Verification items for the finished model (mm, model axes). Face numbers are marked on the shaded views. A direction names the side the tool comes from. Give positions to 0.01 mm unless a question says otherwise; leave off trailing zeros. Order: outer loops, then holes, each group sorted by start corner. A loop starts at its lowest first (then second) coordinate and runs counter-clockwise, first axis right, second up. Notation, with made-up numbers: (8, -12.75) -> (45, -12.75) arc R12 cw to (45, 0.25) -> close; hole circle Ø10 at (-17, -12). An arc over 180 degrees is marked (long way). Return JSON: item names as keys, results as strings. Group by question number.
(1) Cross-section at C-C on y = 67.5. Enter the section's corners in (x, z).
(2) Tool access check on the marked faces 1, 2 and 3. Record the directions out of +Z, -Z, +X, -X, +Y, -Y that give a thin tool (end or side, any length) a straight path to the whole face; none if there is none.
(3) Thickness scan on line 1 along Y through (x, z) = (-35.5, 1.7); line 2 along X through (y, z) = (-35, 2); line 3 along Y through (x, z) = (30, 46). Record the ranges inside material, lowest first.
(4) Cross-section at D-D on x = 35.5. Enter the section's corners in (y, z).
(5) Cross-section at A-A on x = 0. Enter the section's corners in (y, z), then the cut area to 3 significant figures.
(6) Depth check by flat-ended pin: pin 1 Ø4.5 at (x, y) = (-14.5, 64) entering from -Z; pin 2 Ø12 at (x, z) = (11.5, 34.5) entering from +Y; pin 3 Ø6 at (x, y) = (-35.5, 35.5) entering from +Z. Enter the tip coordinate at first touch or a pass-through.
(7) Cross-section at B-B on y = 0. Enter the section's corners in (x, z).
from build123d import *

# Parameters (mm, degrees)
F0_W     = 90
F0_H     = 90
F0_W_2   = 80
F0_H_2   = 80
F0_R     = 2.5
F0_R_2   = 39
F0_H_3   = 10
F1_DEPTH = 5
F0_H_4   = 5
F2_DEPTH = 50
F3_W     = 90
F3_H     = 5
F4_DEPTH = 20
F5_R     = 2.5
F6_DEPTH = 10
F7_SIZE  = 5
F8_SIZE  = 2


with BuildPart() as f1:
    # F0 (on Top) → F1 (new body)
    with BuildSketch(Plane.XY):
        Rectangle(F0_W, F0_H)
        Rectangle(F0_W_2, F0_H_2, mode=Mode.SUBTRACT)
        Rectangle(F0_W_2, F0_H_2)
        with Locations((-35.5, -35.5)):
            Circle(F0_R, mode=Mode.SUBTRACT)
        with Locations((35.5, -35.5)):
            Circle(F0_R, mode=Mode.SUBTRACT)
        Circle(F0_R_2, mode=Mode.SUBTRACT)
        with Locations((-35.5, 35.5)):
            Circle(F0_R, mode=Mode.SUBTRACT)
        with Locations((35.5, 35.5)):
            Circle(F0_R, mode=Mode.SUBTRACT)
        with Locations((0, 50)):
            Rectangle(F0_W, F0_H_3)
    extrude(amount=F1_DEPTH)

    # F0 (on Top) → F2 (join)
    with BuildSketch(Plane.XY):
        with Locations((0, 57.5)):
            Rectangle(F0_W, F0_H_4)
    extrude(amount=F2_DEPTH)

    # F3 (on face) → F4 (join)
    with BuildSketch(Plane.XZ.offset(-55)):
        with Locations((0, 47.5)):
            Rectangle(F3_W, F3_H)
    extrude(amount=-F4_DEPTH)

    # F5 (on face) → F6 (cut)
    with BuildSketch(Plane.XY.offset(50)):
        with Locations((30, 67.5)):
            Circle(F5_R)
        with Locations((-30, 67.5)):
            Circle(F5_R)
    extrude(amount=-F6_DEPTH, mode=Mode.SUBTRACT)

    # F7
    f7_edges = [f1.edges().sort_by_distance(p)[0] for p in [
        (-45, -45, 2.5),
        (45, -45, 2.5),
        (45, 75, 47.5),
        (-45, 75, 47.5),
        (0, 55, 5),
        (0, 60, 0),
    ]]
    chamfer(f7_edges, length=F7_SIZE)

    # F8
    f8_edges = [f1.edges().sort_by_distance(p)[0] for p in [
        (-38, -35.5, 5),
        (33, -35.5, 5),
        (33, 35.5, 5),
        (-38, 35.5, 5),
    ]]
    chamfer(f8_edges, length=F8_SIZE)


solid = f1.part
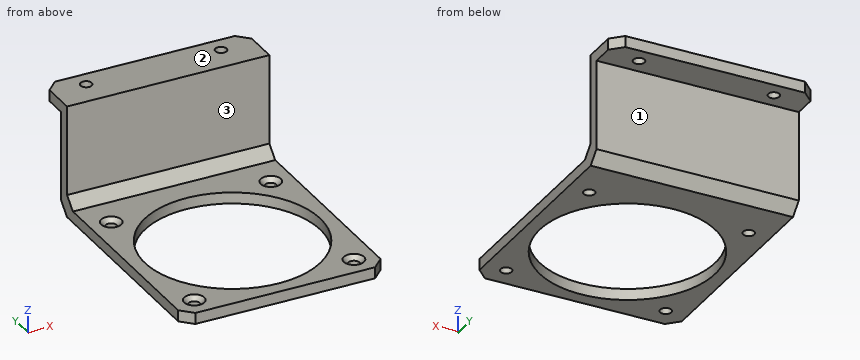
Verdict:
{
 "1": {"outline": "(-45, 45) -> (-32.5, 45) -> (-32.5, 50) -> (-45, 50) -> close; (-27.5, 45) -> (27.5, 45) -> (27.5, 50) -> (-27.5, 50) -> close; (32.5, 45) -> (45, 45) -> (45, 50) -> (32.5, 50) -> close"},
 "2": {"face 1": "-Z, +X, -X, +Y", "face 2": "+Z, +X, -X, +Y, -Y", "face 3": "+Z, +X, -X, -Y"},
 "3": {"line 1": "-45 to -38, -33 to -16.15, 16.15 to 33, 38 to 56.7", "line 2": "-45 to -37.95, -33.05 to -17.2, 17.2 to 33.05, 37.95 to 45", "line 3": "55 to 65, 70 to 75"},
 "4": {"outline": "(-45, 0) -> (-38, 0) -> (-38, 3) -> (-40, 5) -> (-45, 5) -> close; (-33, 0) -> (-16.15, 0) -> (-16.15, 5) -> (-31, 5) -> (-33, 3) -> close; (16.15, 0) -> (33, 0) -> (33, 3) -> (31, 5) -> (16.15, 5) -> close; (38, 0) -> (55, 0) -> (60, 5) -> (60, 45) -> (75, 45) -> (75, 50) -> (55, 50) -> (55, 10) -> (50, 5) -> (40, 5) -> (38, 3) -> close"},
 "5": {"outline": "(-45, 0) -> (-39, 0) -> (-39, 5) -> (-45, 5) -> close; (39, 0) -> (55, 0) -> (60, 5) -> (60, 45) -> (75, 45) -> (75, 50) -> (55, 50) -> (55, 10) -> (50, 5) -> (39, 5) -> close", "area": "435 mm²"},
 "6": {"pin 1": "z = 45", "pin 2": "y = 60", "pin 3": "z = 3.5"},
 "7": {"outline": "(-45, 0) -> (-39, 0) -> (-39, 5) -> (-45, 5) -> close; (39, 0) -> (45, 0) -> (45, 5) -> (39, 5) -> close"}
}
